The listing builds one solid part. Answer for the finished solid, in the listing's coordinates (mm). Face numbers are marked on the shaded views. A direction names the side the tool comes from. Round coordinates to 2 decimals unless told otherwise and drop trailing zeros. Order: outer loops, then holes, each group sorted by start corner. A loop starts at its lowest first (then second) coordinate and runs counter-clockwise, first axis right, second up. Notation, with made-up numbers: (10, 15) - (56, 15) arc R24 ccw to (56, 37) - close; hole circle Ø3 at (31, 53). An arc over 180 degrees is marked (long way). One line per item, written item: value. Start each with the question number.
1. Straight lines are drawn through the part: line 1 (Y direction, x = 30, z = 24); line 2 (X direction, y = 11.75, z = 17); line 3 (X direction, y = 13.5, z = 5). For each, find the intervals that lie inside material, in ascending order.
2. Section A-A, the plane z = 16.5 is taken. Give the vertices of the cut face in (x, y).
3. Section D-D, the plane x = 0 is taken. Give the vertices of the cut face in (y, z), then the cut area to 3 significant figures.
4. Flat-ended cylindrical pins translate along their axes: P1, Ø10, axis at x = 22.5, y = 6, coming from the -Z side; P2, Ø3, axis at x = -13.5, z = 16, coming from the -Y side; P3, Ø2.5, axis at x = 27.43, z = 16.5, coming from the +Y side; P4, Ø2, axis at y = 7, z = 4, coming from the +X side. Find the tip coordinate at first contact, or state that the pin passes through.
5. Section C-C, the plane z = 5 is taken. Give the vertices of the cut face in (x, y).
6. A tool of negligible diameter and unlimited length cuts with its end or side. For the marked faces 1, 2 and 3, from which of +Z, -Z, +X, -X, +Y, -Y can it reach the whole face along a straight path? Write none if from no direction.
7. Section B-B, the plane y = 12.5 is taken. Give the vertices of the cut face in (x, z).
8. For a pull along X with two mould halves and no side action, classify the marked faces 4, 5 and 6 as released by +X, released by -X, zero draft, split by the parting line, or undercut.
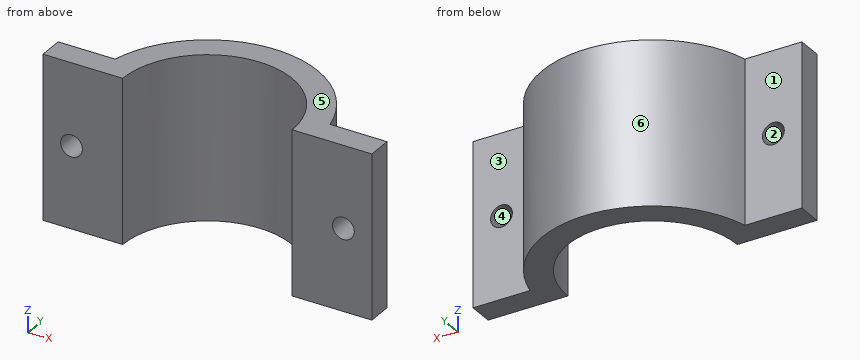
from build123d import *

# Parameters (mm, degrees)
F0_R     = 17.1
F1_DEPTH = 33
F3_D     = 4.4
F5_D     = 4.4
F7_DEPTH = 33


with BuildPart() as f1:
    # F0 (on Top) → F1 (new body)
    with BuildSketch(Plane.XY):
        with BuildLine():
            ThreePointArc((-21.6809247958, -5), (-22.25, 0), (-21.6809247958, 5))
            Line((-21.6809247958, 5), (-33.1809247958, 5))
            Line((-33.1809247958, 5), (-33.1809247958, -5))
            Line((-33.1809247958, -5), (-21.6809247958, -5))
        make_face()
        with BuildLine():
            ThreePointArc((21.6809247958, -5), (22.1072734265, -2.516140228), (22.25, 0))
            ThreePointArc((22.25, 0), (22.1072734265, 2.516140228), (21.6809247958, 5))
            ThreePointArc((21.6809247958, 5), (0, 22.25), (-21.6809247958, 5))
            ThreePointArc((-21.6809247958, 5), (-22.25, 0), (-21.6809247958, -5))
            ThreePointArc((-21.6809247958, -5), (0, -22.25), (21.6809247958, -5))
        make_face()
        Circle(F0_R, mode=Mode.SUBTRACT)
        with BuildLine():
            ThreePointArc((21.6809247958, 5), (22.1072734265, 2.516140228), (22.25, 0))
            ThreePointArc((22.25, 0), (22.1072734265, -2.516140228), (21.6809247958, -5))
            Line((21.6809247958, -5), (33.1809247958, -5))
            Line((33.1809247958, -5), (33.1809247958, 5))
            Line((33.1809247958, 5), (21.6809247958, 5))
        make_face()
    extrude(amount=F1_DEPTH)

    # F3 (through all)
    with Locations(Plane.XZ.offset(5)):
        with Locations((-27.4309247958, 16.5)):
            Hole(F3_D / 2)

    # F5 (through all)
    with Locations(Plane.XZ.offset(5)):
        with Locations((27.4309247958, 16.5)):
            Hole(F5_D / 2)

    # F6 (on face) → F7 (cut)
    with BuildSketch(Plane.XY.offset(33)):
        with BuildLine():
            Line((33.1809247958, 0), (17.1, 0))
            ThreePointArc((17.1, 0), (0, -17.1), (-17.1, 0))
            Line((-17.1, 0), (-33.1809247958, 0))
            Line((-33.1809247958, 0), (-33.1809247958, -5))
            Line((-33.1809247958, -5), (-21.6809247958, -5))
            ThreePointArc((-21.6809247958, -5), (0, -22.25), (21.6809247958, -5))
            Line((21.6809247958, -5), (33.1809247958, -5))
            Line((33.1809247958, -5), (33.1809247958, 0))
        make_face()
        with BuildLine():
            Line((33.1809247958, -22.675672546), (33.1809247958, -5))
            Line((33.1809247958, -5), (21.6809247958, -5))
            ThreePointArc((21.6809247958, -5), (0, -22.25), (-21.6809247958, -5))
            Line((-21.6809247958, -5), (-33.1809247958, -5))
            Line((-33.1809247958, -5), (-33.1809247958, -22.675672546))
            Line((-33.1809247958, -22.675672546), (33.1809247958, -22.675672546))
        make_face()
        with BuildLine():
            ThreePointArc((-17.1, 0), (0, -17.1), (17.1, 0))
            Line((17.1, 0), (-17.1, 0))
        make_face()
    extrude(amount=-F7_DEPTH, mode=Mode.SUBTRACT)


solid = f1.part
Answer list:
1. line 1: y = 0 to 5
1. line 2: x = -18.89 to -12.42, 12.42 to 18.89
1. line 3: x = -17.69 to -10.5, 10.5 to 17.69
2. outline: (-33.18, 0) - (-29.63, 0) - (-29.63, 5) - (-33.18, 5) - close; (-25.23, 0) - (-17.1, 0) arc R17.1 cw to (17.1, 0) - (25.23, 0) - (25.23, 5) - (21.68, 5) arc R22.25 ccw to (-21.68, 5) - (-25.23, 5) - close; (29.63, 0) - (33.18, 0) - (33.18, 5) - (29.63, 5) - close
3. outline: (17.1, 0) - (22.25, 0) - (22.25, 33) - (17.1, 33) - close
3. area: 170 mm²
4. P1: stops at z = 0
4. P2: stops at y = 8.21
4. P3: passes through
4. P4: stops at x = 21.43
5. outline: (-33.18, 0) - (-17.1, 0) arc R17.1 cw to (17.1, 0) - (33.18, 0) - (33.18, 5) - (21.68, 5) arc R22.25 ccw to (-21.68, 5) - (-33.18, 5) - close
6. face 1: +Z, -Z, -X, +Y
6. face 2: +Y, -Y
6. face 3: +Z, -Z, +X, +Y
7. outline: (-18.41, 0) - (-11.67, 0) - (-11.67, 33) - (-18.41, 33) - close; (11.67, 0) - (18.41, 0) - (18.41, 33) - (11.67, 33) - close
8. face 4: undercut
8. face 5: zero draft
8. face 6: split by the parting line
